```python
from build123d import *

# Parameters (mm, degrees)
F1_DEPTH = 15
F2_R     = 10
F4_D     = 2


with BuildPart() as f1:
    # F0 (on Top) → F1 (new body)
    with BuildSketch(Plane.XY):
        with BuildLine():
            Line((-19, 0), (-14, 0))
            ThreePointArc((-14, 0), (-9.899495, 9.899495), (0, 14))
            Line((0, 14), (14.053407, 14))
            Line((14.053407, 14), (14.125915, 33.006928))
            Line((14.125915, 33.006928), (-0.363272, 33.062202))
            Line((-0.363272, 33.062202), (-0.363272, 18.996527))
            ThreePointArc((-0.363272, 18.996527), (-13.562857, 13.305973), (-19, 0))
        make_face()
        with BuildLine():
            ThreePointArc((0, -14), (-9.899495, -9.899495), (-14, 0))
            Line((-14, 0), (-19, 0))
            ThreePointArc((-19, 0), (-13.562857, -13.305973), (-0.363272, -18.996527))
            Line((-0.363272, -18.996527), (-0.363272, -33.062202))
            Line((-0.363272, -33.062202), (14.125915, -33.006928))
            Line((14.125915, -33.006928), (14.053407, -14))
            Line((14.053407, -14), (0, -14))
        make_face()
    extrude(amount=F1_DEPTH)

    # F2
    f2_edges = [f1.edges().sort_by_distance(p)[0] for p in [
        (-0.363272, 18.996527, 7.5),
        (-0.363272, -18.996527, 7.5),
    ]]
    fillet(f2_edges, radius=F2_R)

    # F4 (through all)
    with Locations(Plane(origin=(-0.363272, 0, 0), x_dir=(0, -1, 0), z_dir=(-1, 0, 0))):
        with Locations((-28.308908, 7.5), (28.308908, 7.5)):
            Hole(F4_D / 2)


solid = f1.part
```
CAD build for the part. Positions are in the model's coordinates, mm. A direction names the side the tool comes from. Give positions to 0.01 mm unless a question says otherwise; leave off trailing zeros. Order: outer loops, then holes, each group sorted by start corner. A loop starts at its lowest first (then second) coordinate and runs counter-clockwise, first axis right, second up. Notation, with made-up numbers: M 68.5,-34 L 85.5,-34 A28 cw 85.5,-15 Z; hole C -13.75,2.5 d2. An arc over 180 degrees is marked long. Put each result on its own line as item: value. Start each with the question number.
(1) Mould opens along Y. For faces 1 (the flat face through (7, 14, 7)), 2 (the cylindrical face through (-2.17, -21.35, 7.6)), 3 (the flat face through (1, -14.2, 0)) say: +Y half, -Y half, draft (parallel to the pull), parting line (faces both ways), or undercut.
(2) Saw through at A-A, the plane y = -28.5. Write the cut outline in (x, z), then the cut area to 3 significant figures.
(3) Saw through at B-B, the plane x = -5. Write the cut outline in (y, z) (3 decimals).
(4) Drill centre lines: line 1 along Y through (x, z) = (3.75, 7.5); line 2 along Y through (x, z) = (-10, 8); line 3 along X through (y, z) = (-28, 5.75). Where is each one in solid material? Low to high.
(5) Flat gauge pins, fed straight in: pin 1 Ø1.5 at (y, z) = (5, 10.5) entering from -X; pin 2 Ø3 at (y, z) = (28.31, 7.5) entering from -X; pin 3 Ø12 at (x, y) = (-7, -1) entering from +Z; pin 4 Ø7 at (x, z) = (10, 6) entering from -Y. Where does each tip first touch, or does it go through?
(6) Saw through at D-D, the plane x = 10. Write the cut outline in (y, z), then the cut area to 3 significant figures.
(7) Saw through at C-C, the plane z = 5. Write the cut outline in (x, y).
(8) Which spindle directions (+Z, -Z, +X, -X, +Y, -Y) get a long thin tool onto all of the face, cutting with end or side? Do faces 4 (the flat face through (-0.363, -30, 7)), 5 (the flat face through (7, -14, 7)), 6 (the flat face through (-0.363, 30, 7)), 7 (the cylindrical face through (6.98, 27.31, 7.54)). Say none if no direction does.
Check result:
1. face 1: undercut
1. face 2: -Y half
1. face 3: draft
2. outline: M -0.36,0 L 14.11,0 L 14.11,6.52 L -0.36,6.52 Z; M -0.36,8.48 L 14.11,8.48 L 14.11,15 L -0.36,15 Z
2. area: 189 mm2
3. outline: M -18.645,0 L -13.077,0 L -13.077,15 L -18.645,15 Z; M 13.077,0 L 18.645,0 L 18.645,15 L 13.077,15 Z
4. line 1: y = -33.05 to -29.31, -27.31 to -14, 14 to 27.31, 29.31 to 33.05
4. line 2: y = -16.16 to -9.8, 9.8 to 16.16
4. line 3: x = -0.36 to 14.11
5. pin 1: stops at x = -18.52
5. pin 2: stops at x = -0.37
5. pin 3: passes through
5. pin 4: stops at y = -33.04
6. outline: M -33.02,0 L -14,0 L -14,15 L -33.02,15 Z; M 14,0 L 33.02,0 L 33.02,15 L 14,15 Z; hole C -28.31,7.5 d2; hole C 28.31,7.5 d2
6. area: 564 mm2
7. outline: M -6.79,-17.75 A10 cw -0.36,-27.09 L -0.36,-33.06 L 14.13,-33.01 L 14.05,-14 L 0,-14 A14 cw 0,14 L 14.05,14 L 14.13,33.01 L -0.36,33.06 L -0.36,27.09 A10 cw -6.79,17.75 A19 ccw Z
8. face 4: +Z, -Z, -X, -Y
8. face 5: +Z, -Z, +X
8. face 6: +Z, -Z, -X, +Y
8. face 7: +X, -X
